Could you check a few things on this model? Use its own coordinates, in mm. A direction names the side the tool comes from. Give positions to 0.01 mm unless a question says otherwise; leave off trailing zeros. Order: outer loops, then holes, each group sorted by start corner. A loop starts at its lowest first (then second) coordinate and runs counter-clockwise, first axis right, second up. Notation, with made-up numbers: M 11.5,-27 L 27.5,-27 A21 ccw 27.5,-6 Z; hole C -33,14 d11. An arc over 180 degrees is marked long. Use a Markdown table: item, result. Add a question column.
Item 1: Suppose I cut it at D-D on y = -9. Write out the boundary of the cut face in (x, z), plus the area to 3 significant figures.
Item 2: I'm going to push flat-ended pins straight in: pin 1 Ø10 at (x, y) = (11.5, -9) entering from -Z; pin 2 Ø2.5 at (x, y) = (9, 20.5) entering from -Z; pin 3 Ø1 at (x, y) = (-3.5, -1) entering from -Z. Where does each tip first touch, or does it pass through?
Item 3: If I drill on L1, parallel to Y at x = 20.35, z = -27; L2, parallel to X at y = -16, z = -9.5; L3, parallel to Y at x = 28, z = -27, over which ranges is the centre line in solid material (lowest first)? Write a range as from..to.
Item 4: If we mould it in two halves opening along Y, with no side actions, what happens to faces 1 (the face through (0, -35, -25)), 2 (the face through (0, 19.2, -35)), 3 (the face through (0, -26, -50))? For each: released by +Y, released by -Y, zero draft, split by the parting line, or undercut.
Item 5: Suppose I cut it at B-B on y = 26. Write out the boundary of the cut face in (x, z).
Item 6: For faces 4 (the face through (-1.454, 28.838, -44.495)), 5 (the face through (14.703, 20.017, -0.74)), 6 (the face through (21, -7.9, -7.6)), which set-ups out of +Z, -Z, +X, -X, +Y, -Y let a thin tool reach every point of the face, with its end or its side?
Item 7: Suppose I cut it at C-C on z = -41.7. Count the separate pieces of the cut face and the enclosed holes in it, plus the area to 3 significant figures.
Item 8: Suppose I cut it at A-A on z = -27. Write out the boundary of the cut face in (x, y), plus the area to 3 significant figures.
from build123d import *

# Parameters (mm, degrees)
BOSS_EXTRUDE1_DEPTH = 50
SKETCH5_R           = 3.15
CUT_EXTRUDE2_DEPTH  = 12.5
CUT_EXTRUDE3_DEPTH  = 1.5
SKETCH6_W           = 29
SKETCH6_H           = 3.3
CUT_EXTRUDE4_DEPTH  = 67
SKETCH7_R           = 20
CUT_EXTRUDE5_DEPTH  = 1.5
SKETCH8_R           = 20
CUT_EXTRUDE6_DEPTH  = 1.5


with BuildPart() as part:
    # Sketch1 → Boss-Extrude1 (new body)
    with BuildSketch(Plane.XY):
        Polygon((29, 35), (-29, 35), (0, 4.608), align=None)
        Polygon((-33.5, 30.5), (-33.5, -30.5), (-4.46696193, -0.073376103), align=None)
        Polygon((0, -4.77733119), (-28.7, -35), (28.7, -35), align=None)
        Polygon((4.46696193, -0.073376103), (33.5, -30.5), (33.5, 30.5), align=None)
        Polygon((-4.46696193, -0.073376103), (-33.5, -30.5), (-33.5, -35), (-28.7, -35), (0, -4.77733119), (28.7, -35), (33.5, -35), (33.5, -30.5), (4.46696193, -0.073376103), (33.5, 30.5), (33.5, 35), (29, 35), (0, 4.608), (-29, 35), (-33.5, 35), (-33.5, 30.5), align=None)
    extrude(amount=-BOSS_EXTRUDE1_DEPTH)

    # Sketch5 → Cut-Extrude2 (cut)
    with BuildSketch(Plane(origin=(0, 35, 0), x_dir=(1, 0, 0), z_dir=(0, 1, 0))):
        with Locations(Location((0, 41.7, 0), (0, 0, 180))):
            Circle(SKETCH5_R)
    extrude(amount=-CUT_EXTRUDE2_DEPTH, mode=Mode.SUBTRACT)

    # Sketch1_4 → Cut-Extrude3 (cut)
    with BuildSketch(Plane.XY):
        Polygon((-4.46696193, -0.073376103), (-33.5, -30.5), (-33.5, -35), (-28.7, -35), (0, -4.77733119), (28.7, -35), (33.5, -35), (33.5, -30.5), (4.46696193, -0.073376103), (33.5, 30.5), (33.5, 35), (29, 35), (0, 4.608), (-29, 35), (-33.5, 35), (-33.5, 30.5), align=None)
    extrude(amount=-CUT_EXTRUDE3_DEPTH, mode=Mode.SUBTRACT)

    # Sketch6 → Cut-Extrude4 (cut)
    with BuildSketch(Plane(origin=(33.5, 0, 0), x_dir=(0, 0, -1), z_dir=(1, 0, 0))):
        with Locations((35.5, 20.85)):
            Rectangle(SKETCH6_W, SKETCH6_H)
        with BuildLine():
            Line((50, 0.2), (44.150602701, 0.176602411))
            ThreePointArc((44.150602701, 0.176602411), (8.01471599, -7.252342947), (43.454482672, -17.5))
            Line((43.454482672, -17.5), (50, -17.5))
            Line((50, -17.5), (50, 0.2))
        make_face()
    extrude(amount=-CUT_EXTRUDE4_DEPTH, mode=Mode.SUBTRACT)

    # Sketch7 → Cut-Extrude5 (cut)
    with BuildSketch(Plane(origin=(21, 0, 0), x_dir=(0, 0, -1), z_dir=(1, 0, 0))):
        with Locations((27, -8)):
            Circle(SKETCH7_R)
    extrude(amount=-CUT_EXTRUDE5_DEPTH, mode=Mode.SUBTRACT)

    # Sketch8 → Cut-Extrude6 (cut)
    with BuildSketch(Plane(origin=(-22.5, 0, 0), x_dir=(0, 0, -1), z_dir=(1, 0, 0))):
        with Locations((27, -8)):
            Circle(SKETCH8_R)
    extrude(amount=-CUT_EXTRUDE6_DEPTH, mode=Mode.SUBTRACT)


solid = part.part
Findings below:
| question | item | result |
|---|---|---|
| 1 | outline | M -33.5,-8.03 L -24,-8.03 L -24,-7.03 L -22.5,-7.03 L -22.5,-8.03 L 19.5,-8.03 L 19.5,-7.03 L 21,-7.03 L 21,-8.03 L 33.5,-8.03 L 33.5,0 L 12.98,0 L 12.98,-1.5 L 4.01,-1.5 L 4.01,0 L -4.01,0 L -4.01,-1.5 L -12.98,-1.5 L -12.98,0 L -33.5,0 Z |
| 1 | area | 508 mm^2 |
| 2 | pin 1 | stops at z = -8.97 |
| 2 | pin 2 | stops at z = -21 |
| 2 | pin 3 | stops at z = -9.54 |
| 3 | L1 | y = -35..-28, 12..19.2, 22.5..35 |
| 3 | L2 | x = -33.5..-24, -22.5..19.5, 21..33.5 |
| 3 | L3 | y = -35..-27, 11..19.2, 22.5..35 |
| 4 | face 1 | released by -Y |
| 4 | face 2 | undercut |
| 4 | face 3 | zero draft |
| 5 | outline | M -33.5,-50 L 33.5,-50 L 33.5,0 L 29.23,0 L 29.23,-1.5 L 20.41,-1.5 L 20.41,0 L -20.41,0 L -20.41,-1.5 L -29.23,-1.5 L -29.23,0 L -33.5,0 Z; hole C 0,-41.7 d6.3 |
| 6 | face 4 | +Y |
| 6 | face 5 | +Z |
| 6 | face 6 | none |
| 7 | separate pieces | 4 |
| 7 | enclosed holes | 0 |
| 7 | area | 2,770 mm^2 |
| 8 | outline | M -33.5,-35 L 33.5,-35 L 33.5,-27 L 21,-27 L 21,-28 L 19.5,-28 L 19.5,-27 L -22.5,-27 L -22.5,-28 L -24,-28 L -24,-27 L -33.5,-27 Z; M -33.5,11 L -24,11 L -24,12 L -22.5,12 L -22.5,11 L 19.5,11 L 19.5,12 L 21,12 L 21,11 L 33.5,11 L 33.5,19.2 L -33.5,19.2 Z; M -33.5,22.5 L 33.5,22.5 L 33.5,35 L -33.5,35 Z |
| 8 | area | 1,920 mm^2 |
